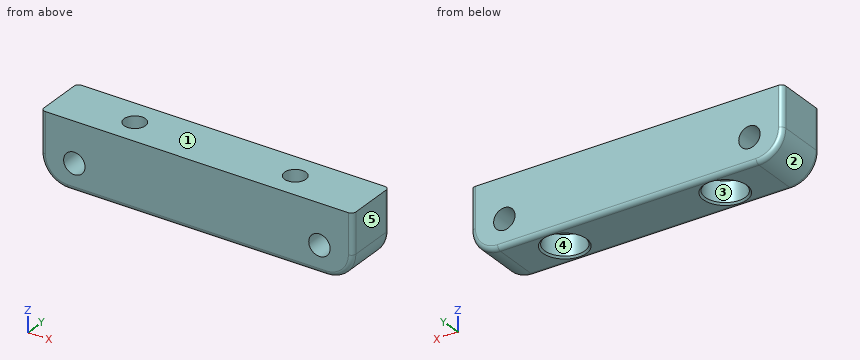
from build123d import *

# Parameters (mm, degrees)
SKETCH2_W           = 70
SKETCH2_H           = 15
SKETCH2_R           = 2.4
BOSS_EXTRUDE1_DEPTH = 6
SKETCH4_R           = 2.4
CUT_EXTRUDE1_DEPTH  = 39.548670535
FILLET1_R           = 6
FILLET2_R           = 1
SKETCH5_R           = 4.5
CUT_EXTRUDE2_DEPTH  = 5
CHAMFER1_SIZE       = 0.4


with BuildPart() as part:
    # Sketch2 → Boss-Extrude1 (new, symmetric)
    with BuildSketch(Plane(origin=(0, 0, 0), x_dir=(1, 0, 0), z_dir=(0, 1, 0))):
        Rectangle(SKETCH2_W, SKETCH2_H)
        with Locations(Location((-27.5, 1.5, 0), (0, 0, 270))):
            Circle(SKETCH2_R, mode=Mode.SUBTRACT)
        with Locations(Location((27.5, 1.5, 0), (0, 0, 90))):
            Circle(SKETCH2_R, mode=Mode.SUBTRACT)
    extrude(amount=BOSS_EXTRUDE1_DEPTH, both=True)

    # Sketch4 → Cut-Extrude1 (cut, through all)
    with BuildSketch(Plane.XY.offset(7.5)):
        with Locations((-18, 0)):
            Circle(SKETCH4_R)
        with Locations(Location((18, 0, 0), (0, 0, 180))):
            Circle(SKETCH4_R)
    extrude(amount=-CUT_EXTRUDE1_DEPTH, mode=Mode.SUBTRACT)

    # Fillet1
    fillet1_edges = [part.edges().sort_by_distance(p)[0] for p in [
        (-35, 0, -7.5),
        (35, 0, -7.5),
    ]]
    fillet(fillet1_edges, radius=FILLET1_R)

    # Fillet2
    fillet2_edges = [part.edges().sort_by_distance(p)[0] for p in [
        (35, 6, 3),
        (-35, -6, 3),
        (-35, 6, 3),
        (0, -6, -7.5),
        (33.242640687, -6, -5.742640687),
        (-33.242640687, -6, -5.742640687),
        (0, 6, -7.5),
        (33.242640687, 6, -5.742640687),
        (-33.242640687, 6, -5.742640687),
        (35, -6, 3),
    ]]
    fillet(fillet2_edges, radius=FILLET2_R)

    # Sketch5 → Cut-Extrude2 (cut)
    with BuildSketch(Plane(origin=(0, 0, -7.5), x_dir=(-1, 0, 0), z_dir=(0, 0, -1))):
        with Locations((-18, 0)):
            Circle(SKETCH5_R)
        with Locations((18, 0)):
            Circle(SKETCH5_R)
    extrude(amount=-CUT_EXTRUDE2_DEPTH, mode=Mode.SUBTRACT)

    # Chamfer1
    chamfer1_edges = [part.edges().sort_by_distance(p)[0] for p in [
        (22.5, 0, -7.5),
        (-13.5, 0, -7.5),
    ]]
    chamfer(chamfer1_edges, length=CHAMFER1_SIZE)


solid = part.part
Geometry check sheet. Reference: the model listing, model coordinates, mm. Face numbers are marked on the shaded views. A direction names the side the tool comes from. Coordinates: 2 decimals unless noted, no trailing zeros. Order: outer loops, then holes, each group sorted by start corner. A loop starts at its lowest first (then second) coordinate and runs counter-clockwise, first axis right, second up. Notation, with made-up numbers: (45, 40.25) - (100, 40.25) arc R19 ccw to (100, 66.25) - close; hole circle Ø3 at (-16.75, 69.25). An arc over 180 degrees is marked (long way). Answer in a Markdown table with one row per item. Add a question column.
1) Cross-section at C-C, the plane x = -27.5. Record the cut outline in (y, z), then the cut area to 3 significant figures.
2) Set-up check for the marked faces 4 and 5: record each of +Z, -Z, +X, -X, +Y, -Y from which the full face is reachable in a straight line by a thin tool's end or side.
3) Cross-section at A-A, the plane y = 0. Record the cut outline in (x, z), then the cut area to 3 significant figures.
4) Cross-section at B-B, the plane z = -0.5. Record the cut outline in (x, y).
5) Release check for a two-part mould opening along X. For the marked faces 1, 2 and 3 record: +X half, -X half, draft (parallel to the pull), parting line (faces both ways), or undercut.
6) Cross-section at D-D, the plane z = 2.5. Record the cut outline in (x, y), then the cut area to 3 significant figures.
7) Material ranges on line 1 along Z through (x, y) = (27.5, -1.75); line 2 along Y through (x, z) = (18, 1.75); line 3 along Y through (x, z) = (18, -4.55), recorded low to high. Write a range as [from, to].
8) Gauge pin test, flat end, axial feed: P1, Ø1.5, axis at y = 3.5, z = -6, coming from the -X side. Record the tip position at first contact, or that the pin passes through.
Check result:
| question | item | result |
|---|---|---|
| 1 | outline | (-6, -6.5) arc R1 ccw to (-5, -7.5) - (5, -7.5) arc R1 ccw to (6, -6.5) - (6, -3.9) - (-6, -3.9) - close; (-6, 0.9) - (6, 0.9) - (6, 7.5) - (-6, 7.5) - close |
| 1 | area | 122 mm² |
| 2 | face 4 | -Z |
| 2 | face 5 | +Z, -Z, +X, +Y, -Y |
| 3 | outline | (-35, -1.5) arc R6 ccw to (-29, -7.5) - (-22.9, -7.5) - (-22.5, -7.1) - (-22.5, -2.5) - (-20.4, -2.5) - (-20.4, 7.5) - (-35, 7.5) - close; (-15.6, -2.5) - (-13.5, -2.5) - (-13.5, -7.1) - (-13.1, -7.5) - (13.1, -7.5) - (13.5, -7.1) - (13.5, -2.5) - (15.6, -2.5) - (15.6, 7.5) - (-15.6, 7.5) - close; (20.4, -2.5) - (22.5, -2.5) - (22.5, -7.1) - (22.9, -7.5) - (29, -7.5) arc R6 ccw to (35, -1.5) - (35, 7.5) - (20.4, 7.5) - close; hole circle Ø4.8 at (-27.5, -1.5); hole circle Ø4.8 at (27.5, -1.5) |
| 3 | area | 812 mm² |
| 4 | outline | (-35, -5) arc R1 ccw to (-34, -6) - (-29.68, -6) - (-29.68, 6) - (-34, 6) arc R1 ccw to (-35, 5) - close; (-25.32, -6) - (25.32, -6) - (25.32, 6) - (-25.32, 6) - close; (29.68, -6) - (34, -6) arc R1 ccw to (35, -5) - (35, 5) arc R1 ccw to (34, 6) - (29.68, 6) - close; hole circle Ø4.8 at (-18, 0); hole circle Ø4.8 at (18, 0) |
| 5 | face 1 | draft |
| 5 | face 2 | -X half |
| 5 | face 3 | undercut |
| 6 | outline | (-35, -5) arc R1 ccw to (-34, -6) - (34, -6) arc R1 ccw to (35, -5) - (35, 5) arc R1 ccw to (34, 6) - (-34, 6) arc R1 ccw to (-35, 5) - close; hole circle Ø4.8 at (-18, 0); hole circle Ø4.8 at (18, 0) |
| 6 | area | 803 mm² |
| 7 | line 1 | z = [-7.5, -3.9], [0.9, 7.5] |
| 7 | line 2 | y = [-6, -2.4], [2.4, 6] |
| 7 | line 3 | y = [-6, -4.5], [4.5, 6] |
| 8 | P1 | stops at x = -33.68 |
